Part print with two shaded views. Sizes in mm from the minimum x, y, z corner. A direction names the side the tool comes from. Round coordinates to 2 decimals unless told otherwise and drop trailing zeros. Write each loop counter-clockwise with the first axis right and the second up, starting at its lowest first coordinate (ties: lowest second). Pieces come first, ordered by that corner, then holes. Notation, with made-up numbers: (80, -31.5) -> (111, -31.5) arc R30 cw to (111, -9.5) -> close; hole circle Ø4 at (25, -17.75). An arc over 180 degrees is marked (long way). Answer in a Markdown table with one row per item.
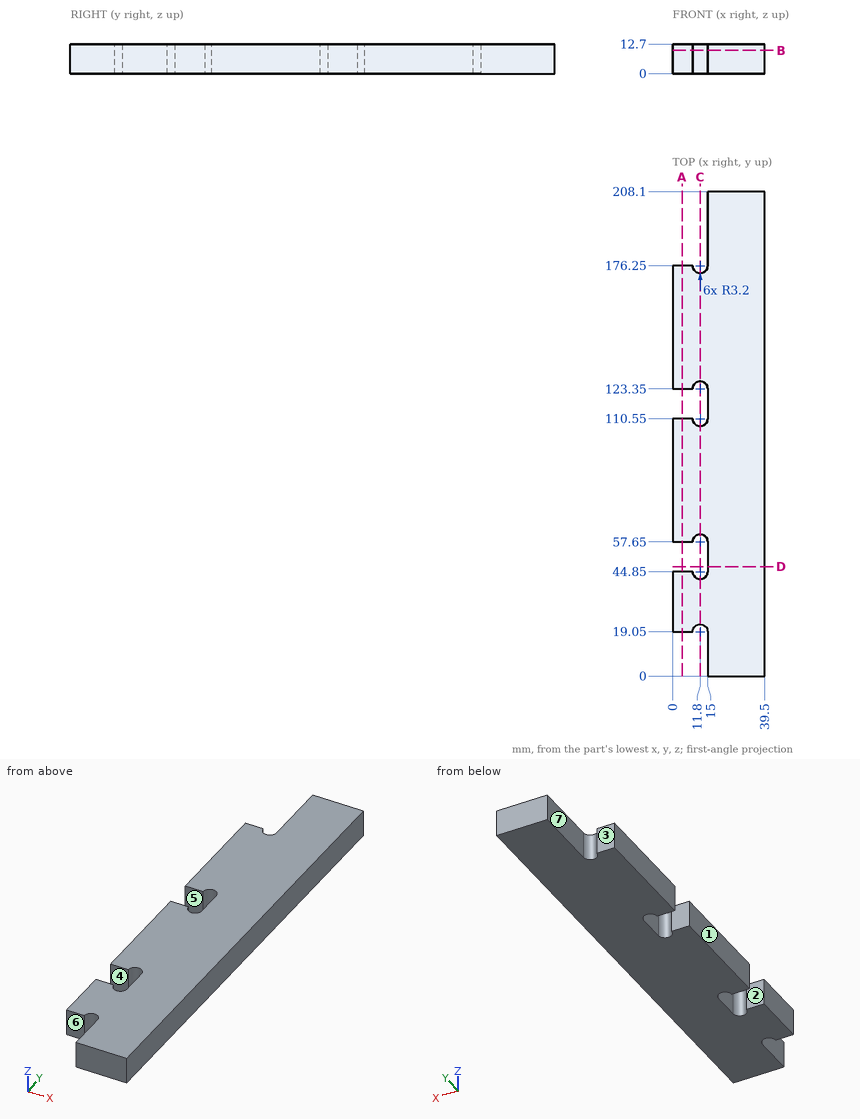
Q1. Saw through at B-B on z = 10. Write the cut outline in (x, y).
A:
| item | result |
|---|---|
| outline | (0, 19.05) -> (8.6, 19.05) arc R3.2 cw to (15, 19.05) -> (15, 0) -> (39.5, 0) -> (39.5, 208.1) -> (15, 208.1) -> (15, 176.25) arc R3.2 cw to (8.6, 176.25) -> (0, 176.25) -> (0, 123.35) -> (8.6, 123.35) arc R3.2 cw to (15, 123.35) -> (15, 110.55) arc R3.2 cw to (8.6, 110.55) -> (0, 110.55) -> (0, 57.65) -> (8.6, 57.65) arc R3.2 cw to (15, 57.65) -> (15, 44.85) arc R3.2 cw to (8.6, 44.85) -> (0, 44.85) -> close |
Q2. Saw through at A-A on x = 4. Write the cut outline in (y, z), plus the area to 3 significant figures.
A:
| item | result |
|---|---|
| outline | (19.05, 0) -> (44.85, 0) -> (44.85, 12.7) -> (19.05, 12.7) -> close; (57.65, 0) -> (110.55, 0) -> (110.55, 12.7) -> (57.65, 12.7) -> close; (123.35, 0) -> (176.25, 0) -> (176.25, 12.7) -> (123.35, 12.7) -> close |
| area | 1,670 mm² |
Q3. Saw through at D-D on y = 47. Write the cut outline in (x, z).
A:
| item | result |
|---|---|
| outline | (15, 0) -> (39.5, 0) -> (39.5, 12.7) -> (15, 12.7) -> close |
Q4. Drop flat-ended pins along their axis: P1, Ø4, axis at y = 199, z = 8, coming from the -X side; P2, Ø4.5, axis at x = 2.5, z = 9.5, coming from the +Y side; P3, Ø7, axis at x = 4.5, z = 8, coming from the -Y side. Give the stop position or say it passes through.
A:
| item | result |
|---|---|
| P1 | x = 15 |
| P2 | y = 176.25 |
| P3 | y = 19.05 |
Q5. Which spindle directions (+Z, -Z, +X, -X, +Y, -Y) get a long thin tool onto all of the face, cutting with end or side? Do the marked faces 5, 6 and 7. Say none if no direction does.
A:
| item | result |
|---|---|
| face 5 | +Z, -Z, -X |
| face 6 | +Z, -Z, -X, -Y |
| face 7 | +Z, -Z, -X, +Y |
Q6. Wall check: line 1 (Y direction, x = 8.5, z = 8.25); line 2 (Y direction, x = 10.5, z = 8.25); line 3 (X direction, y = 112, z = 8.5). Give the ranges that are in metal, low to high. Write a range as [from, to].
A:
| item | result |
|---|---|
| line 1 | [19.05, 44.85], [57.65, 110.55], [123.35, 176.25] |
| line 2 | [21.97, 41.93], [60.57, 107.63], [126.27, 173.33] |
| line 3 | [15, 39.5] |
Q7. Saw through at C-C on x = 11.8. Write the cut outline in (y, z).
A:
| item | result |
|---|---|
| outline | (22.25, 0) -> (41.65, 0) -> (41.65, 12.7) -> (22.25, 12.7) -> close; (60.85, 0) -> (107.35, 0) -> (107.35, 12.7) -> (60.85, 12.7) -> close; (126.55, 0) -> (173.05, 0) -> (173.05, 12.7) -> (126.55, 12.7) -> close |
Q8. Two-plate mould, pull along Y, no slides. Class the marked faces 1, 2, 3 and 4: released by +Y, released by -Y, zero draft, split by the parting line, or undercut.
A:
| item | result |
|---|---|
| face 1 | zero draft |
| face 2 | undercut |
| face 3 | released by +Y |
| face 4 | undercut |
